from build123d import *

# Parameters (mm, degrees)
BOX004_W          = 10
BOX004_H          = 14
BOX004_DEPTH      = 10
BOX006_W          = 10
BOX006_H          = 2.7
BOX006_DEPTH      = 10
BOX003_W          = 10
BOX003_H          = 14
BOX003_DEPTH      = 10
CYLINDER_R        = 1.35
CYLINDER_DEPTH    = 10
BOX005_W          = 10
BOX005_H          = 2.7
BOX005_DEPTH      = 10
CYLINDER001_R     = 1.35
CYLINDER001_DEPTH = 10
BOX007_W          = 10
BOX007_H          = 5
BOX007_DEPTH      = 10
BOX008_W          = 10
BOX008_H          = 5
BOX008_DEPTH      = 10
BOX002_W          = 115.7
BOX002_H          = 10.2
BOX002_DEPTH      = 7
BOX_W             = 132
BOX_H             = 12.5
BOX_DEPTH         = 10
BOX001_W          = 118
BOX001_H          = 10.2
BOX001_DEPTH      = 5
CHAMFER_SIZE      = 0.5


with BuildPart() as box004:
    # Box004 → Box004 (new body)
    with BuildSketch(Plane(origin=(118, -2, 10), x_dir=(1, 0, 0), z_dir=(0, 0, 1))):
        with Locations((5, 7)):
            Rectangle(BOX004_W, BOX004_H)
    extrude(amount=BOX004_DEPTH)


with BuildPart() as box006:
    # Box006 → Box006 (new body)
    with BuildSketch(Plane(origin=(121.5, 3.76, 0), x_dir=(1, 0, 0), z_dir=(0, 0, 1))):
        with Locations((5, 1.35)):
            Rectangle(BOX006_W, BOX006_H)
    extrude(amount=BOX006_DEPTH)


with BuildPart() as box003:
    # Box003 → Box003 (new body)
    with BuildSketch(Plane(origin=(-10, -2, 10), x_dir=(1, 0, 0), z_dir=(0, 0, 1))):
        with Locations((5, 7)):
            Rectangle(BOX003_W, BOX003_H)
    extrude(amount=BOX003_DEPTH)


with BuildPart() as cylinder:
    # Cylinder → Cylinder (new body)
    with BuildSketch(Plane(origin=(-3.5, 5.1, 0), x_dir=(1, 0, 0), z_dir=(0, 0, 1))):
        Circle(CYLINDER_R)
    extrude(amount=CYLINDER_DEPTH)


with BuildPart() as box005:
    # Box005 → Box005 (new body)
    with BuildSketch(Plane(origin=(-13.3, 3.76, 0), x_dir=(1, 0, 0), z_dir=(0, 0, 1))):
        with Locations((5, 1.35)):
            Rectangle(BOX005_W, BOX005_H)
    extrude(amount=BOX005_DEPTH)


with BuildPart() as cylinder001:
    # Cylinder001 → Cylinder001 (new body)
    with BuildSketch(Plane(origin=(121.5, 5.1, 0), x_dir=(1, 0, 0), z_dir=(0, 0, 1))):
        Circle(CYLINDER001_R)
    extrude(amount=CYLINDER001_DEPTH)


with BuildPart() as box007:
    # Box007 → Box007 (new body)
    with BuildSketch(Plane(origin=(-11, 2.6, 8), x_dir=(1, 0, 0), z_dir=(0, 0, 1))):
        with Locations((5, 2.5)):
            Rectangle(BOX007_W, BOX007_H)
    extrude(amount=BOX007_DEPTH)


with BuildPart() as box008:
    # Box008 → Box008 (new body)
    with BuildSketch(Plane(origin=(119, 2.6, 8), x_dir=(1, 0, 0), z_dir=(0, 0, 1))):
        with Locations((5, 2.5)):
            Rectangle(BOX008_W, BOX008_H)
    extrude(amount=BOX008_DEPTH)


with BuildPart() as fusion:
    # Box002 → Box002 (new body)
    with BuildSketch(Plane(origin=(1.15, 0, 8), x_dir=(1, 0, 0), z_dir=(0, 0, 1))):
        with Locations((57.85, 5.1)):
            Rectangle(BOX002_W, BOX002_H)
    extrude(amount=BOX002_DEPTH)

    # Fusion: union Box004, Box006, Box003, Cylinder, Box005, Cylinder001, Box007, Box008
    add(box004.part)
    add(box006.part)
    add(box003.part)
    add(cylinder.part)
    add(box005.part)
    add(cylinder001.part)
    add(box007.part)
    add(box008.part)


with BuildPart() as box:
    # Box → Box (new body)
    with BuildSketch(Plane(origin=(-7, -1.15, 5), x_dir=(1, 0, 0), z_dir=(0, 0, 1))):
        with Locations((66, 6.25)):
            Rectangle(BOX_W, BOX_H)
    extrude(amount=BOX_DEPTH)


with BuildPart() as chamfer_body:
    # Box001 → Box001 (new body)
    with BuildSketch(Plane.XY):
        with Locations((59, 5.1)):
            Rectangle(BOX001_W, BOX001_H)
    extrude(amount=BOX001_DEPTH)

    # Fusion001: union Box
    add(box.part)

    # Cut: cut Fusion
    add(fusion.part, mode=Mode.SUBTRACT)

    # Chamfer
    chamfer_edges = [chamfer_body.edges().sort_by_distance(p)[0] for p in [
        (1.15, 5.1, 15),
        (59, 0, 15),
        (116.85, 5.1, 15),
        (59, 10.2, 15),
    ]]
    chamfer(chamfer_edges, length=CHAMFER_SIZE)


solid = chamfer_body.part
Verification items for the finished model (mm, model axes). A direction names the side the tool comes from. Coordinates: 2 decimals unless noted, no trailing zeros. Write each loop counter-clockwise with the first axis right and the second up, starting at its lowest first coordinate (ties: lowest second). Pieces come first, ordered by that corner, then holes. Notation, with made-up numbers: M 27.5,34 L 54.5,34 A29 cw 54.5,61 Z; hole C -9,6.5 d6. An arc over 180 degrees is marked long. Use a Markdown table: item, result.
Q1. Thickness scan on line 1 (Y direction, x = 4, z = 10.5); line 2 (X direction, y = 1.5, z = 11); line 3 (Z direction, x = 25, y = 5.25). Record the ranges inside material, lowest first.
Reply:
| item | result |
|---|---|
| line 1 | y = -1.15 to 0, 10.2 to 11.35 |
| line 2 | x = 0 to 1.15, 116.85 to 118 |
| line 3 | z = 0 to 8 |
Q2. Sectioned sample at C-C, the plane x = 52.5. Record the boundary of the cut face in (y, z), plus the area to 3 significant figures.
Reply:
| item | result |
|---|---|
| outline | M -1.15,5 L 0,5 L 0,0 L 10.2,0 L 10.2,5 L 11.35,5 L 11.35,15 L 10.7,15 L 10.2,14.5 L 10.2,8 L 0,8 L 0,14.5 L -0.5,15 L -1.15,15 Z |
| area | 104 mm² |
Q3. Sectioned sample at A-A, the plane z = 11.5. Record the boundary of the cut face in (x, y).
Reply:
| item | result |
|---|---|
| outline | M 0,-1.15 L 118,-1.15 L 118,11.35 L 0,11.35 Z; hole M 1.15,0 L 116.85,0 L 116.85,10.2 L 1.15,10.2 Z |
Q4. Set-up check for faces 1 (the face through (-4, 8, 10)), 2 (the face through (120, 5, 8)), 3 (the face through (58, 0, 11)), 4 (the face through (118, 5, 2)), 5 (the face through (58, 10.2, 2)): record each of +Z, -Z, +X, -X, +Y, -Y from which the full face is reachable in a straight line by a thin tool's end or side.
Reply:
| item | result |
|---|---|
| face 1 | +Z, -X, +Y, -Y |
| face 2 | +Z, +X |
| face 3 | +Z |
| face 4 | -Z, +X, +Y, -Y |
| face 5 | -Z, +X, -X, +Y |
Q5. Sectioned sample at B-B, the plane y = 5.1. Record the boundary of the cut face in (x, z), plus the area to 3 significant figures.
Reply:
| item | result |
|---|---|
| outline | M -2.15,5 L 0,5 L 0,0 L 118,0 L 118,5 L 120.15,5 L 120.15,8 L 119,8 L 119,10 L 118,10 L 118,15 L 117.35,15 L 116.85,14.5 L 116.85,8 L 1.15,8 L 1.15,14.5 L 0.65,15 L 0,15 L 0,10 L -1,10 L -1,8 L -2.15,8 Z |
| area | 977 mm² |
Q6. Go/stop test with flat-tipped pins: P1, Ø4, axis at x = 123, y = 5.5, coming from the +Z side; P2, Ø2, axis at x = 27.5, z = 3.5, coming from the +Y side; P3, Ø1.5, axis at y = 5, z = 1.5, coming from the -X side. Record where each tip stops, or that it passes through.
Reply:
| item | result |
|---|---|
| P1 | stops at z = 8 |
| P2 | stops at y = 10.2 |
| P3 | stops at x = 0 |
Q7. Draft check along Y on faces 6 (the face through (118, 5, 12)), 7 (the face through (-5, 6.46, 6)), 8 (the face through (58, -1.15, 10)). Enter one of: +Y half, -Y half, draft (parallel to the pull), parting line (faces both ways), or undercut.
Reply:
| item | result |
|---|---|
| face 6 | draft |
| face 7 | undercut |
| face 8 | -Y half |
